from build123d import *

# Parameters (mm, degrees)
SKETCH1_W                      = 30
SKETCH1_H                      = 93
BASE_FLANGE1_DEPTH             = 3.175
EDGE_FLANGE1_STRIP_W           = 20.32
EDGE_FLANGE1_STRIP_H           = 3.175
EDGE_FLANGE1_STRIP_CUT_DEPTH   = 30
EDGE_FLANGE1_STRIP_2_W         = 20.32
EDGE_FLANGE1_STRIP_2_H         = 3.175
EDGE_FLANGE1_STRIP_CUT_2_DEPTH = 30
EDGE_FLANGE1_DEPTH             = 30
EDGE_FLANGE1_BEND_DEPTH        = 30
CUT_EXTRUDE1_DEPTH             = 65.316449101
CUT_EXTRUDE1_DEPTH_BACK        = 65.316449101
SKETCH12_OUTSIDE_W             = 54.33
SKETCH12_OUTSIDE_H             = 65.505
SKETCH12_OUTSIDE_R             = 1.35
SKETCH12_OUTSIDE_R_2           = 5.25


# Sheet-metal steps are written as plain solids
with BuildPart() as part:
    # Sketch1 → Base-Flange1 (new body)
    with BuildSketch(Plane(origin=(0, 0, 0), x_dir=(1, 0, 0), z_dir=(0, 1, 0))):
        Rectangle(SKETCH1_W, SKETCH1_H)
    extrude(amount=BASE_FLANGE1_DEPTH)

    # Edge-Flange1 strip (across the edge) → Edge-Flange1 strip cut (cut)
    with BuildSketch(Plane(origin=(15, 0, 46.5), x_dir=(0, 0, -1), z_dir=(-1, 0, 0))):
        with Locations((-6.35, -1.5875)):
            Rectangle(EDGE_FLANGE1_STRIP_W, EDGE_FLANGE1_STRIP_H)
    extrude(amount=EDGE_FLANGE1_STRIP_CUT_DEPTH, mode=Mode.SUBTRACT)

    # Edge-Flange1 strip 2 (across the edge) → Edge-Flange1 strip cut 2 (cut)
    with BuildSketch(Plane(origin=(-15, 0, -46.5), x_dir=(0, 0, 1), z_dir=(1, 0, 0))):
        with Locations((-6.35, -1.5875)):
            Rectangle(EDGE_FLANGE1_STRIP_2_W, EDGE_FLANGE1_STRIP_2_H)
    extrude(amount=EDGE_FLANGE1_STRIP_CUT_2_DEPTH, mode=Mode.SUBTRACT)

    # Edge-Flange1 section (across the edge) → Edge-Flange1 (add)
    with BuildSketch(Plane(origin=(15, 0, 46.5), x_dir=(0, 0, -1), z_dir=(-1, 0, 0))):
        with BuildLine():
            Line((-3.175, 3.81), (-3.175, 38))
            Line((-3.175, 38), (0, 38))
            Line((0, 38), (0, 3.81))
            ThreePointArc((0, 3.81), (1.115923164, 1.115923164), (3.81, 0))
            Line((3.81, 0), (3.81, -3.175))
            ThreePointArc((3.81, -3.175), (-1.129140867, -1.129140867), (-3.175, 3.81))
        make_face()
    extrude(amount=EDGE_FLANGE1_DEPTH)

    # Edge-Flange1 section 2 (across the edge) → Edge-Flange1 bend (add)
    with BuildSketch(Plane(origin=(-15, 0, -46.5), x_dir=(0, 0, 1), z_dir=(1, 0, 0))):
        with BuildLine():
            Line((-3.175, 3.81), (-3.175, 38))
            Line((-3.175, 38), (0, 38))
            Line((0, 38), (0, 3.81))
            ThreePointArc((0, 3.81), (1.115923164, 1.115923164), (3.81, 0))
            Line((3.81, 0), (3.81, -3.175))
            ThreePointArc((3.81, -3.175), (-1.129140867, -1.129140867), (-3.175, 3.81))
        make_face()
    extrude(amount=EDGE_FLANGE1_BEND_DEPTH)

    # Sketch12 outside → Cut-Extrude1 (cut, two sides: drawn at the far end of the back side and taken through both)
    # profile 1 of 10: a face of its own
    with BuildSketch(Plane.XY.offset(-CUT_EXTRUDE1_DEPTH_BACK)):
        with Locations((0, -17.4125)):
            Rectangle(SKETCH12_OUTSIDE_W, SKETCH12_OUTSIDE_H)
        with BuildLine():
            Line((12.945561693, -26.188458018), (15, -3.81))
            Line((15, -3.81), (15, 3.175))
            Line((15, 3.175), (-15, 3.175))
            Line((-15, 3.175), (-15, -3.81))
            Line((-15, -3.81), (-12.945561693, -26.188458018))
            ThreePointArc((-12.945561693, -26.188458018), (0, -38), (12.945561693, -26.188458018))
        make_face(mode=Mode.SUBTRACT)
    # profile 2 of 10: a face of its own
    with BuildSketch(Plane.XY.offset(-CUT_EXTRUDE1_DEPTH_BACK)):
        with Locations((0, -36)):
            Circle(SKETCH12_OUTSIDE_R)
    # profile 3 of 10: a face of its own
    with BuildSketch(Plane.XY.offset(-CUT_EXTRUDE1_DEPTH_BACK)):
        with Locations((-7.778174593, -32.778174593)):
            Circle(SKETCH12_OUTSIDE_R)
    # profile 4 of 10: a face of its own
    with BuildSketch(Plane.XY.offset(-CUT_EXTRUDE1_DEPTH_BACK)):
        with Locations((-11, -25)):
            Circle(SKETCH12_OUTSIDE_R)
    # profile 5 of 10: a face of its own
    with BuildSketch(Plane.XY.offset(-CUT_EXTRUDE1_DEPTH_BACK)):
        with Locations((-7.778174593, -17.221825407)):
            Circle(SKETCH12_OUTSIDE_R)
    # profile 6 of 10: a face of its own
    with BuildSketch(Plane.XY.offset(-CUT_EXTRUDE1_DEPTH_BACK)):
        with Locations((0, -14)):
            Circle(SKETCH12_OUTSIDE_R)
    # profile 7 of 10: a face of its own
    with BuildSketch(Plane.XY.offset(-CUT_EXTRUDE1_DEPTH_BACK)):
        with Locations((7.778174593, -17.221825407)):
            Circle(SKETCH12_OUTSIDE_R)
    # profile 8 of 10: a face of its own
    with BuildSketch(Plane.XY.offset(-CUT_EXTRUDE1_DEPTH_BACK)):
        with Locations((11, -25)):
            Circle(SKETCH12_OUTSIDE_R)
    # profile 9 of 10: a face of its own
    with BuildSketch(Plane.XY.offset(-CUT_EXTRUDE1_DEPTH_BACK)):
        with Locations((7.778174593, -32.778174593)):
            Circle(SKETCH12_OUTSIDE_R)
    # profile 10 of 10: a face of its own
    with BuildSketch(Plane.XY.offset(-CUT_EXTRUDE1_DEPTH_BACK)):
        with Locations((0, -25)):
            Circle(SKETCH12_OUTSIDE_R_2)
    extrude(amount=CUT_EXTRUDE1_DEPTH + CUT_EXTRUDE1_DEPTH_BACK, mode=Mode.SUBTRACT)


solid = part.part
Here's how the part is built. I have some questions about the finished solid (model axes, mm). A direction names the side the tool comes from. Coordinates: 2 decimals unless noted, no trailing zeros. Order: outer loops, then holes, each group sorted by start corner. A loop starts at its lowest first (then second) coordinate and runs counter-clockwise, first axis right, second up.
Item 1: For faces 1 (the face through (7.6, -31.44, -48.11)), 2 (the face through (-0.21, -1.146, -45.414)), which set-ups out of +Z, -Z, +X, -X, +Y, -Y let a thin tool reach every point of the face, with its end or its side?
Result sheet:
face 1: +Z, -Z
face 2: +X, -X, -Y
Item 2: If we section it at C-C on y = -25: State how many separate pieces and enclosed holes the cut face has, plus the area to 3 significant figures.
Result sheet:
separate pieces: 8
enclosed holes: 0
area: 64.8 mm2
Item 3: I need wall thicknesses on line 1 (Z direction, x = 10.5, y = -30) (3 decimals); line 2 (X direction, y = -25, z = 48.1); line 3 (Y direction, x = 0, z = 47.6). Which ranges of each line are inside material? Lowest first, please.
Result sheet:
line 1: z = -49.675 to -46.5, 46.5 to 49.675
line 2: x = -13.05 to -12.35, -9.65 to -5.25, 5.25 to 9.65, 12.35 to 13.05
line 3: y = -38 to -37.35, -34.65 to -30.25, -19.75 to -15.35, -12.65 to 1.16
Item 4: If we mould it in two halves opening along Y, with no side actions, what happens to faces 3 (the face through (0, -38, -48)), 4 (the face through (0, 3.175, -1)), 5 (the face through (-0.29, -37.32, -48.11))? For each: +Y half, -Y half, draft (parallel to the pull), parting line (faces both ways), or undercut.
Result sheet:
face 3: -Y half
face 4: +Y half
face 5: undercut
Item 5: For P1, Ø10, axis at x = 5, z = -29, coming from the -Y side, with a flat end and sliding along its axis, tell me the tip position at first contact or that it passes through.
Result sheet:
P1: stops at y = 0
Item 6: If we section it at A-A on x = 11: List the corners of the cut face in (y, z) for me (3 decimals), plus the area to 3 significant figures.
Result sheet:
outline: (-31.928, -49.675) - (-26.35, -49.675) - (-26.35, -46.5) - (-31.928, -46.5) - close; (-31.928, 46.5) - (-26.35, 46.5) - (-26.35, 49.675) - (-31.928, 49.675) - close; (-23.65, -49.675) - (-3.81, -49.675) arc R6.985 ccw to (3.175, -42.69) - (3.175, 42.69) arc R6.985 ccw to (-3.81, 49.675) - (-23.65, 49.675) - (-23.65, 46.5) - (-3.81, 46.5) arc R3.81 cw to (0, 42.69) - (0, -42.69) arc R3.81 cw to (-3.81, -46.5) - (-23.65, -46.5) - close
area: 486 mm2
Item 7: If we section it at B-B on y = -14: List the corners of the cut face in (x, z) for me (3 decimals), plus the area to 3 significant figures.
Result sheet:
outline: (-14.065, -49.675) - (-1.35, -49.675) - (-1.35, -46.5) - (-14.065, -46.5) - close; (-14.065, 46.5) - (-1.35, 46.5) - (-1.35, 49.675) - (-14.065, 49.675) - close; (1.35, -49.675) - (14.065, -49.675) - (14.065, -46.5) - (1.35, -46.5) - close; (1.35, 46.5) - (14.065, 46.5) - (14.065, 49.675) - (1.35, 49.675) - close
area: 161 mm2
